Design review of the part built by this model. Coordinates are the model's own, in mm. A direction names the side the tool comes from. Round coordinates to 2 decimals unless told otherwise and drop trailing zeros. Loops run counter-clockwise (first coordinate to the right, second up) from the corner with the lowest first, then second, coordinate; pieces in that order, holes last. Notation, with made-up numbers: (-17, -39) - (-12, -39) arc R22 cw to (-12, -32) - close; hole circle Ø3 at (45.25, -26). An arc over 180 degrees is marked (long way). Return JSON: item names as keys, results as strings. Group by question number.
(1) For faces 1 (the flat face through (6, 3.216, 7)), 2 (the flat face through (-13, 8.89, 7)), list the 3-axis set-ups (+Z, -Z, +X, -X, +Y, -Y) from which the entire face can be reached by the end or side of a thin tool; tool diameter is ignored.
(2) We need section B-B, the plane x = -5. Write out the cut boundary in (y, z), and give its area (3 significant figures).
(3) We need section A-A, the plane z = 7. Write out the cut boundary in (x, y) (1 decimal).
(4) Wall thickness on L1, parallel to Y at x = -20, z = 2.5; L2, parallel to Y at x = -2, z = 11.25; L3, parallel to X at y = 5.5, z = 6: over which ranges is each line inside the solid? List them lowest first. Write a range as [from, to].
(5) Clearance check with flat-ended pins moving along their axes: pin 1 (4 mm diameter, centred on x = -15, z = 8.5, fed in from -Y); pin 2 (4 mm diameter, centred on y = 5.5, z = 8, fed in from -X). State where each tip first meets the part, or that it passes through.
(6) We need section C-C, the plane y = 8.5. Write out the cut boundary in (x, z).
Autodesk Inventor part; units mm, degrees
ref_plane "YZ Plane" through (0, 0, 0) normal (1, 0, 0) x (0, 1, 0)
ref_plane "XZ Plane" through (0, 0, 0) normal (0, 1, 0) x (-1, 0, 0)
ref_plane "XY Plane" through (0, 0, 0) normal (0, 0, 1) x (1, 0, 0)
sketch "Sketch1" plane through (0, 0, 0) normal (0, 0, 1) x (1, 0, 0)
  arc A0 (5.1036, 3.2163) -> (2.772, 5.3579) centre (0, 0) ccw
  arc A1 (13.6525, 7.62) -> (6.7446, 3.2163) centre (13.6525, 0) ccw
  line L0 (13.6525, 11.43) -> (0, 11.43)
  line L1 (-20.955, 11.43) -> (0, 11.43)
  line L2 (5.1036, 3.2163) -> (6.7446, 3.2163)
  line L3 (-20.955, 11.43) -> (-20.955, 8.89)
  line L4 (-20.955, 8.89) -> (-4.055, 8.89)
  line L5 (-4.055, 8.89) -> (2.772, 5.3579)
  line L6 (13.6525, 7.62) -> (13.6525, 11.43)
  dimension "d0" = 12.065
  dimension "d4" = 2.54
extrude "Extrusion1" add sketch "Sketch1" along normal blind 13.97
sketch "Sketch2" plane through (5.1036, 3.2163, 0) normal (0, -1, 0) x (1, 0, 0)
  point P0 (-5.1036, 0)
properties part number "Antibuckler"
Solutions:
{
 "1": {"face 1": "+Z, -Z, +X, -X, -Y", "face 2": "+Z, -Z, -X, -Y"},
 "2": {"outline": "(8.89, 0) - (11.43, 0) - (11.43, 13.97) - (8.89, 13.97) - close", "area": "35.5 mm^2"},
 "3": {"outline": "(-21, 8.9) - (-4.1, 8.9) - (2.8, 5.4) arc R6 cw to (5.1, 3.2) - (6.7, 3.2) arc R7.6 cw to (13.7, 7.6) - (13.7, 11.4) - (-21, 11.4) - close"},
 "4": {"L1": "[8.89, 11.43]", "L2": "[7.83, 11.43]", "L3": "[2.5, 8.38]"},
 "5": {"pin 1": "y = 8.89", "pin 2": "x = -1.37"},
 "6": {"outline": "(-3.3, 0) - (13.65, 0) - (13.65, 13.97) - (-3.3, 13.97) - close"}
}
